The listing builds one solid part. Answer for the finished solid, in the listing's coordinates (mm). Round coordinates to 2 decimals unless told otherwise and drop trailing zeros. Write each loop counter-clockwise with the first axis right and the second up, starting at its lowest first coordinate (ties: lowest second). Pieces come first, ordered by that corner, then holes. Notation, with made-up numbers: (63, 89) - (86, 89) arc R21 ccw to (86, 118) - close; hole circle Ø11 at (-35.75, -31.5). An arc over 180 degrees is marked (long way). Use a Markdown table: item, result. Add a question column.
1) Each of these flat-tipped pins is pushed along its axis until it touches: P1, Ø7.5, axis at x = 245, y = -67.5, coming from the +Z side; P2, Ø5, axis at x = 214.5, z = -4, coming from the +Y side. Where does it stop, or does it pass through?
2) A cutting plane is placed at B-B (x = -204.5). Give the vertices of the cut face in (y, z), then the cut area to 3 significant figures.
3) Find the intervals of material crossed by probe 1 along Y at (x, z) = (245, -6.25); probe 2 along X at (y, z) = (87.5, -6); probe 3 along X at (y, z) = (65, -6), in increasing order. Write a range as from..to.
4) A cutting plane is placed at A-A (z = -1.5). Give the vertices of the cut face in (x, y).
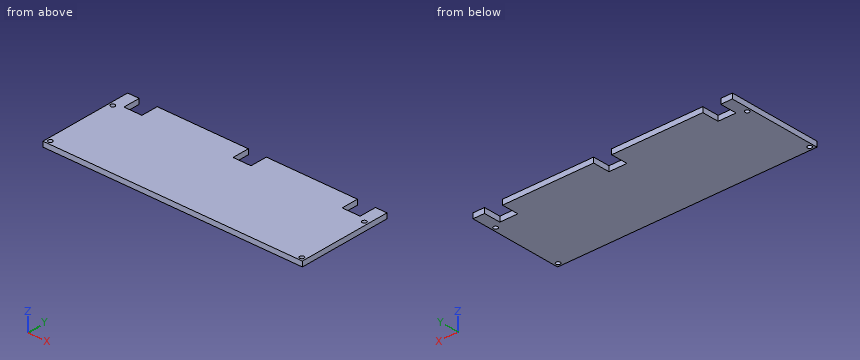
```python
from build123d import *

# Parameters (mm, degrees)
IZIM1_W               = 505
IZIM1_H               = 150
TABAN_FLAN_1_DEPTH    = 10
IZIM2_R               = 4.25
KES_EKSTR_ZYON1_DEPTH = 10
IZIM3_W               = 22.5
IZIM3_H               = 33
IZIM3_W_2             = 177.5
SEKME1_DEPTH          = 10


# Sheet-metal steps are written as plain solids
with BuildPart() as part:
    # Çizim1 → Taban-Flanş1 (new body)
    with BuildSketch(Plane.XY):
        Rectangle(IZIM1_W, IZIM1_H)
    extrude(amount=-TABAN_FLAN_1_DEPTH)

    # Çizim2 → Kes-Ekstrüzyon1 (cut)
    with BuildSketch(Plane.XY):
        with Locations((-245, 67.5)):
            Circle(IZIM2_R)
        with Locations(Location((245, 67.5, 0), (0, 0, 180))):
            Circle(IZIM2_R)
    kes_ekstr_zyon1 = extrude(amount=-KES_EKSTR_ZYON1_DEPTH, mode=Mode.SUBTRACT)

    # Aynalama1: Kes-Ekstrüzyon1 across plane
    add(kes_ekstr_zyon1.mirror(Plane.ZX), mode=Mode.SUBTRACT)

    # Çizim3 → Sekme1 (add)
    with BuildSketch(Plane.XY):
        with Locations((241.25, 91.5)):
            Rectangle(IZIM3_W, IZIM3_H)
        with Locations((106.25, 91.5)):
            Rectangle(IZIM3_W_2, IZIM3_H)
        with Locations((-106.25, 91.5)):
            Rectangle(IZIM3_W_2, IZIM3_H)
        with Locations((-241.25, 91.5)):
            Rectangle(IZIM3_W, IZIM3_H)
    extrude(amount=-SEKME1_DEPTH)


solid = part.part
```
Entries:
| question | item | result |
|---|---|---|
| 1 | P1 | passes through |
| 1 | P2 | stops at y = 75 |
| 2 | outline | (-75, -10) - (75, -10) - (75, 0) - (-75, 0) - close |
| 2 | area | 1,500 mm² |
| 3 | probe 1 | y = -75..-71.75, -63.25..63.25, 71.75..108 |
| 3 | probe 2 | x = -252.5..-230, -195..-17.5, 17.5..195, 230..252.5 |
| 3 | probe 3 | x = -252.5..-248.44, -241.56..241.56, 248.44..252.5 |
| 4 | outline | (-252.5, -75) - (252.5, -75) - (252.5, 108) - (230, 108) - (230, 75) - (195, 75) - (195, 108) - (17.5, 108) - (17.5, 75) - (-17.5, 75) - (-17.5, 108) - (-195, 108) - (-195, 75) - (-230, 75) - (-230, 108) - (-252.5, 108) - close; hole circle Ø8.5 at (-245, -67.5); hole circle Ø8.5 at (-245, 67.5); hole circle Ø8.5 at (245, -67.5); hole circle Ø8.5 at (245, 67.5) |
